```python
from build123d import *

# Parameters (mm, degrees)
MODEL_R             = 1.5
MODEL_R_2           = 2.4892
BOSS_EXTRUDE1_DEPTH = 3.175


with BuildPart() as part:
    # Model → Boss-Extrude1 (new body)
    with BuildSketch(Plane.XY):
        with BuildLine():
            Line((323.667245607, 226.12499065), (349.307245607, 226.12499065))
            ThreePointArc((349.307245607, 226.12499065), (358.287501728, 222.405246771), (362.007245607, 213.42499065))
            Line((362.007245607, 213.42499065), (362.007245607, 162.55499065))
            Line((362.007245607, 162.55499065), (440.597245607, 162.55499065))
            Line((440.597245607, 162.55499065), (440.597245607, 310.17499065))
            Line((440.597245607, 310.17499065), (410.434211887, 310.17499065))
            Line((410.434211887, 310.17499065), (410.434211887, 301.91999065))
            ThreePointArc((410.434211887, 301.91999065), (408.20236556, 296.531836978), (402.814211887, 294.29999065))
            Line((402.814211887, 294.29999065), (353.054686067, 294.29999065))
            ThreePointArc((353.054686067, 294.29999065), (347.666532395, 296.531836978), (345.434686067, 301.91999065))
            Line((345.434686067, 301.91999065), (345.434686067, 310.17499065))
            Line((345.434686067, 310.17499065), (290.913803272, 310.17499065))
            Line((290.913803272, 310.17499065), (290.913803272, 301.91999065))
            ThreePointArc((290.913803272, 301.91999065), (288.681956945, 296.531836978), (283.293803272, 294.29999065))
            Line((283.293803272, 294.29999065), (195.647245607, 294.29999065))
            Line((195.647245607, 294.29999065), (195.647245607, 226.12499065))
            Line((195.647245607, 226.12499065), (223.137245607, 226.12499065))
            ThreePointArc((223.137245607, 226.12499065), (228.525399279, 223.893144323), (230.757245607, 218.50499065))
            Line((230.757245607, 218.50499065), (230.757245607, 162.55499065))
            Line((230.757245607, 162.55499065), (310.967245607, 162.55499065))
            Line((310.967245607, 162.55499065), (310.967245607, 213.42499065))
            ThreePointArc((310.967245607, 213.42499065), (314.686989486, 222.405246771), (323.667245607, 226.12499065))
        make_face()
        with Locations((303.347245607, 167.55499065)):
            Circle(MODEL_R, mode=Mode.SUBTRACT)
        with Locations((434.597245607, 167.55499065)):
            Circle(MODEL_R, mode=Mode.SUBTRACT)
        with Locations((218.347245607, 272.55499065)):
            Circle(MODEL_R, mode=Mode.SUBTRACT)
        with Locations((317.989745607, 239.93349065)):
            Circle(MODEL_R_2, mode=Mode.SUBTRACT)
        with Locations((303.702245607, 260.57099065)):
            Circle(MODEL_R_2, mode=Mode.SUBTRACT)
        with Locations((317.989745607, 281.20849065)):
            Circle(MODEL_R_2, mode=Mode.SUBTRACT)
        with Locations((303.347245607, 302.55499065)):
            Circle(MODEL_R, mode=Mode.SUBTRACT)
        with Locations((332.277245607, 260.57099065)):
            Circle(MODEL_R_2, mode=Mode.SUBTRACT)
        with Locations((349.597245607, 272.55499065)):
            Circle(MODEL_R, mode=Mode.SUBTRACT)
        with Locations((434.597245607, 302.55499065)):
            Circle(MODEL_R, mode=Mode.SUBTRACT)
    extrude(amount=BOSS_EXTRUDE1_DEPTH)


solid = part.part
```
Geometry: final body of the model. Coordinates: model frame, mm. A direction names the side the tool comes from. Round coordinates to 2 decimals unless told otherwise and drop trailing zeros. Loops run counter-clockwise (first coordinate to the right, second up) from the corner with the lowest first, then second, coordinate; pieces in that order, holes last.
Item 1: Line query: L1, parallel to X at y = 203, z = 1.2; L2, parallel to Y at x = 319, z = 1.75 (3 decimals); L3, parallel to X at y = 273.5, z = 1.6. Output: solid intervals per line, ascending.
Checked values:
L1: x = 230.76 to 310.97, 362.01 to 440.6
L2: y = 225.236 to 237.659, 242.208 to 278.934, 283.483 to 310.175
L3: x = 195.65 to 217.18, 219.51 to 348.43, 350.76 to 440.6
Item 2: Section C-C, the plane x = 390. Output: boundary loops of the cut face in (y, z) (3 decimals).
Checked values:
outline: (162.555, 0) - (294.3, 0) - (294.3, 3.175) - (162.555, 3.175) - close
Item 3: Reachability of faces 1 (the cylindrical face through (408.26, 296.59, 1.57)), 2 (the cylindrical face through (314.59, 222.31, 1.57)), 3 (the cylindrical face through (316.014, 279.694, 1.565)) from +Z, -Z, +X, -X, +Y, -Y: full face, straight path, thin tool, end or side. Return the list, or none.
Checked values:
face 1: +Z, -Z, +Y
face 2: +Z, -Z, -Y
face 3: +Z, -Z
Item 4: Contact query for flat-ended pins moving along their axis: P1, Ø2.5, axis at x = 434.6, y = 167.55, coming from the +Z side; P2, Ø1.6, axis at x = 369, z = 1.5, coming from the +Y side; P3, Ø8, axis at x = 317.99, y = 239.93, coming from the -Z side; P4, Ø1, axis at y = 180.5, z = 1.5, coming from the -X side. Output: stop coordinate, or through.
Checked values:
P1: passes through
P2: stops at y = 294.3
P3: stops at z = 0
P4: stops at x = 230.76
Item 5: Section B-B, the plane z = 1.2. State how many separate pieces and enclosed holes the cut face has, plus the area to 3 significant figures.
Checked values:
separate pieces: 1
enclosed holes: 10
area: 28,100 mm2
Item 6: Section A-A, the plane y = 174. Output: boundary loops of the cut face in (x, z) (3 decimals), plus the area to 3 significant figures.
Checked values:
outline: (230.757, 0) - (310.967, 0) - (310.967, 3.175) - (230.757, 3.175) - close; (362.007, 0) - (440.597, 0) - (440.597, 3.175) - (362.007, 3.175) - close
area: 504 mm2
Item 7: Section D-D, the plane y = 223. Output: boundary loops of the cut face in (x, z) (3 decimals), plus the area to 3 significant figures.
Checked values:
outline: (229.29, 0) - (315.324, 0) - (315.324, 3.175) - (229.29, 3.175) - close; (357.65, 0) - (440.597, 0) - (440.597, 3.175) - (357.65, 3.175) - close
area: 537 mm2
Item 8: Mould query, pull axis X, two halves, no side actions, for faces 4 (the flat face through (316, 237, 0)), 5 (the cylindrical face through (316.16, 241.62, 1.57)), 6 (the cylindrical face through (228.47, 223.95, 1.57)). Classes: released by +X, released by -X, zero draft, split by the parting line, or undercut.
Checked values:
face 4: zero draft
face 5: undercut
face 6: released by -X
